from build123d import *

# Parameters (mm, degrees)
BOSS_EXTRUDE1_DEPTH     = 1
SKETCH2_W               = 2.1
SKETCH2_H               = 1.8
CUT_EXTRUDE1_DEPTH      = 1
CUT_EXTRUDE1_DEPTH_BACK = 2
FILLET1_R               = 0.5
SKETCH3_R               = 0.5
SKETCH3_R_2             = 0.975
CUT_EXTRUDE2_DEPTH      = 1
CUT_EXTRUDE2_DEPTH_BACK = 2


with BuildPart() as part:
    # Sketch1 → Boss-Extrude1 (new body)
    with BuildSketch(Plane(origin=(0, 0, 0), x_dir=(1, 0, 0), z_dir=(0, 1, 0))):
        with BuildLine():
            Line((0, -1), (0, -21.45))
            ThreePointArc((0, -21.45), (0.219669914, -21.980330086), (0.75, -22.2))
            Line((0.75, -22.2), (0.75, -29.3))
            ThreePointArc((0.75, -29.3), (1.189339828, -30.360660172), (2.25, -30.8))
            Line((2.25, -30.8), (48.75, -30.8))
            ThreePointArc((48.75, -30.8), (49.810660172, -30.360660172), (50.25, -29.3))
            Line((50.25, -29.3), (50.25, -22.2))
            ThreePointArc((50.25, -22.2), (50.780330086, -21.980330086), (51, -21.45))
            Line((51, -21.45), (51, -1))
            ThreePointArc((51, -1), (50.707106781, -0.292893219), (50, 0))
            Line((50, 0), (1, 0))
            ThreePointArc((1, 0), (0.292893219, -0.292893219), (0, -1))
        make_face()
    extrude(amount=BOSS_EXTRUDE1_DEPTH)

    # Sketch2 → Cut-Extrude1 (cut, two sides)
    with BuildSketch(Plane(origin=(0, 1, 0), x_dir=(1, 0, 0), z_dir=(0, 1, 0))) as cut_extrude1_sk:
        with Locations((1.05, -13.35)):
            Rectangle(SKETCH2_W, SKETCH2_H)
        with BuildLine():
            Line((29.6, 0), (21.4, 0))
            ThreePointArc((21.4, 0), (22.107106781, -0.292893219), (22.4, -1))
            ThreePointArc((22.4, -1), (25.5, -4.1), (28.6, -1))
            ThreePointArc((28.6, -1), (28.892893219, -0.292893219), (29.6, 0))
        make_face()
        with Locations((49.95, -11.65)):
            Rectangle(SKETCH2_W, SKETCH2_H)
    extrude(amount=CUT_EXTRUDE1_DEPTH, mode=Mode.SUBTRACT)
    extrude(cut_extrude1_sk.sketch, amount=-CUT_EXTRUDE1_DEPTH_BACK, mode=Mode.SUBTRACT)

    # Fillet1
    fillet1_edges = [part.edges().sort_by_distance(p)[0] for p in [
        (0, 0.5, 14.25),
        (0, 0.5, 12.45),
        (51, 0.5, 10.75),
        (51, 0.5, 12.55),
    ]]
    fillet(fillet1_edges, radius=FILLET1_R)

    # Sketch3 → Cut-Extrude2 (cut, two sides)
    with BuildSketch(Plane(origin=(0, 1, 0), x_dir=(1, 0, 0), z_dir=(0, 1, 0))) as cut_extrude2_sk:
        with Locations((3.52, -3.45)):
            Circle(SKETCH3_R)
        with Locations((20.2, -3.45)):
            Circle(SKETCH3_R)
        with Locations((38.3, -2.25)):
            Circle(SKETCH3_R)
        with Locations((47.14, -2.25)):
            Circle(SKETCH3_R)
        with Locations((48.627, -20.91)):
            Circle(SKETCH3_R_2)
        with Locations((45.29, -19.95)):
            Circle(SKETCH3_R)
        with Locations((27.94, -19.95)):
            Circle(SKETCH3_R)
        with Locations((20.29, -19.95)):
            Circle(SKETCH3_R)
        with Locations((9.75, -19.43)):
            Circle(SKETCH3_R)
    extrude(amount=CUT_EXTRUDE2_DEPTH, mode=Mode.SUBTRACT)
    extrude(cut_extrude2_sk.sketch, amount=-CUT_EXTRUDE2_DEPTH_BACK, mode=Mode.SUBTRACT)


solid = part.part
Input: part model. Units: mm. Frame: model coordinates. A direction names the side the tool comes from. Coordinates: 2 decimals unless noted, no trailing zeros. Loops run counter-clockwise (first coordinate to the right, second up) from the corner with the lowest first, then second, coordinate; pieces in that order, holes last. Notation, with made-up numbers: (-18.75, -13) -> (31.25, -13) arc R21 ccw to (31.25, 8) -> close; hole circle Ø8 at (34, -26.75). An arc over 180 degrees is marked (long way). Write each question's results on one line, items separated by ' | '. Start each with the question number.
Q1. Section C-C, the plane y = 0.7. State how many separate pieces and enclosed holes the cut face has, plus the area to 3 significant figures.
Q2. Pin query (flat end, axial travel): pin 1 (0.5 mm diameter, centred on x = 1, y = 0.5, fed in from +Z); pin 2 (1.8 mm diameter, centred on x = 48.627, z = 20.91, fed in from -Y). Return the tip coordinate at first contact, or that it passes through.
Q3. Pull-direction query (X, two-part tool) for faces 1 (the flat face through (0, 0.5, 6.4)), 2 (the cylindrical face through (19.831, 0.507, 3.112)), 3 (the flat face through (25.2, 0.5, 30.8)); classes: released by +X, released by -X, zero draft, split by the parting line, or undercut.
Q4. Section A-A, the plane x = 45.29. Return the cut outline in (y, z).
Q5. Reachability of faces 4 (the cylindrical face through (22.099, 0.507, 0.285)), 5 (the flat face through (0.75, 0.5, 25.7)), 6 (the flat face through (2.1, 0.5, 13.4)) from +Z, -Z, +X, -X, +Y, -Y: full face, straight path, thin tool, end or side. Return the list, or none.
Q6. Ray query, line 1 (X direction, y = 0.45, z = 3.45); line 2 (Z direction, x = 45.29, y = 0.5); line 3 (X direction, y = 0.15, z = 11). Return the intervals inside material, ascending. Write a range as from..to.
Q7. Section B-B, the plane z = 2.25. Return the cut outline in (x, y), plus the area to 3 significant figures.
Q8. Section D-D, the plane x = 27.94. Return the cut outline in (y, z).
Found:
1) separate pieces: 1 | enclosed holes: 9 | area: 1,520 mm2
2) pin 1: z = 30.42 | pin 2: through
3) face 1: released by -X | face 2: undercut | face 3: zero draft
4) outline: (0, 0) -> (1, 0) -> (1, 19.45) -> (0, 19.45) -> close; (0, 20.45) -> (1, 20.45) -> (1, 30.8) -> (0, 30.8) -> close
5) face 4: -Z, +Y, -Y | face 5: +Z, -X, +Y, -Y | face 6: -X, +Y, -Y
6) line 1: 0..3.02, 4.02..19.7, 20.7..23.6, 27.4..51 | line 2: 0..19.45, 20.45..30.8 | line 3: 0..48.9
7) outline: (0, 0) -> (22.66, 0) -> (22.66, 1) -> (0, 1) -> close; (28.34, 0) -> (37.8, 0) -> (37.8, 1) -> (28.34, 1) -> close; (38.8, 0) -> (46.64, 0) -> (46.64, 1) -> (38.8, 1) -> close; (47.64, 0) -> (51, 0) -> (51, 1) -> (47.64, 1) -> close | area: 43.3 mm2
8) outline: (0, 2.91) -> (1, 2.91) -> (1, 19.45) -> (0, 19.45) -> close; (0, 20.45) -> (1, 20.45) -> (1, 30.8) -> (0, 30.8) -> close
